Could you check a few things on this model? Use its own coordinates, in mm. A direction names the side the tool comes from. Give positions to 0.01 mm unless a question says otherwise; leave off trailing zeros. Write each loop counter-clockwise with the first axis right and the second up, starting at its lowest first coordinate (ties: lowest second). Pieces come first, ordered by that corner, then holes. Notation, with made-up numbers: (27, 71) -> (82, 71) arc R19 ccw to (82, 90) -> close; hole circle Ø5 at (-35, 45.5). An arc over 180 degrees is marked (long way). One line per question, with ' | ' between items.
from build123d import *

# Parameters (mm, degrees)
ESQUISSE1_W                                  = 4.2
ESQUISSE1_H                                  = 3
ESQUISSE1_W_2                                = 5
ESQUISSE1_H_2                                = 9.7
D_GAGEMENT_M31_D                             = 3.4
ESQUISSE4_W                                  = 1.25
ESQUISSE4_H                                  = 12.7
TROU_POUR_TARAUDAGE_POUR_TROU_TARAUD_2_COUNT = 2
TROU_POUR_TARAUDAGE_POUR_TROU_TARAUD_2_PITCH = 4.6


with BuildPart() as part:
    # Esquisse1 → Révolution1 (revolve)
    with BuildSketch(Plane.XY, mode=Mode.PRIVATE) as r_volution1_sk:
        with Locations((-2.1, 4.5)):
            Rectangle(ESQUISSE1_W, ESQUISSE1_H)
        with Locations((2.5, 7.85)):
            Rectangle(ESQUISSE1_W_2, ESQUISSE1_H_2)
    revolve(r_volution1_sk.sketch.rotate(Axis((0, 0, 0), (1, 0, 0)), 90), axis=Axis((0, 0, 0), (1, 0, 0)))

    # Dégagement M31 (through all)
    with Locations(Plane.ZY):
        with Locations((4.75, 8.227241336), (-4.75, 8.227241336), (-9.5, 0), (-4.75, -8.227241336), (4.75, -8.227241336), (9.5, 0)):
            Hole(D_GAGEMENT_M31_D / 2)

    # Esquisse4 → Trou pour taraudage pour trou taraudé M3x0.51 (revolve, cut)
    with BuildSketch(Plane(origin=(2.5, 0, 0), x_dir=(0, 0, -1), z_dir=(1, 0, 0))):
        with Locations((0.625, 6.35)):
            Rectangle(ESQUISSE4_W, ESQUISSE4_H)
    trou_pour_taraudage_pour_trou_taraud_m3 = revolve(axis=Axis((2.5, -6.35, 0), (0, 1, 0)), mode=Mode.SUBTRACT)

    # Trou pour taraudage pour trou taraud 2: Trou pour taraudage pour trou taraudé M3x0.51 ×2
    with Locations(*[(-i * TROU_POUR_TARAUDAGE_POUR_TROU_TARAUD_2_PITCH, 0, 0) for i in range(1, TROU_POUR_TARAUDAGE_POUR_TROU_TARAUD_2_COUNT)]):
        add(trou_pour_taraudage_pour_trou_taraud_m3, mode=Mode.SUBTRACT)


solid = part.part
Q1. Imagine slicing it at B-B on z = 0. Please give me the cut outline in (x, y), and give its area (4 significant figures).
Answer below:
outline: (-4.2, -6) -> (0, -6) -> (0, -12.7) -> (5, -12.7) -> (5, -3) -> (-4.2, -3) -> close; (-4.2, 3) -> (-3.35, 3) -> (-3.35, 6) -> (-4.2, 6) -> close; (-0.85, 3) -> (1.25, 3) -> (1.25, 12.7) -> (0, 12.7) -> (0, 6) -> (-0.85, 6) -> close; (3.75, 3) -> (5, 3) -> (5, 12.7) -> (3.75, 12.7) -> close | area: 90.45 mm^2
Q2. Will these pins go through, and if not, where does the flat tip stop? pin 1 (1 mm diameter, centred on y = 9.5, z = -2.5, fed in from -X); pin 2 (5 mm diameter, centred on x = 2, y = 7.5, fed in from +Z); pin 3 (2 mm diameter, centred on x = -2.1, z = 0, fed in from +Y); pin 4 (2 mm diameter, centred on y = 8.23, z = 4.75, fed in from -X).
Answer below:
pin 1: stops at x = 0 | pin 2: stops at z = 11.67 | pin 3: stops at y = -2.83 | pin 4: passes through
Q3. Imagine slicing it at C-C on z = -9.5. Please give me the cut outline in (x, y), and give its area (3 significant figures).
Answer below:
outline: (0, -8.43) -> (5, -8.43) -> (5, -1.7) -> (0, -1.7) -> close; (0, 1.7) -> (5, 1.7) -> (5, 8.43) -> (0, 8.43) -> close | area: 67.3 mm^2
Q4. If we mould it in two halves opening along Y, with no side actions, what happens to faces 4 (the cylindrical face through (2.5, 7.7, -10.1)), 5 (the flat face through (-4.2, -3, -1)), 6 (the cylindrical face through (2.5, 6.7, 4))? For each: +Y half, -Y half, draft (parallel to the pull), parting line (faces both ways), or undercut.
Answer below:
face 4: parting line | face 5: draft | face 6: undercut
Q5. If I drill on line 1 along Z through (x, y) = (4, -8); line 2 along Y through (x, z) = (3.4, -4.75); line 3 along Y through (x, z) = (4.25, 6.25), over which ranges is the centre line in solid material (lowest first)?
Answer below:
line 1: z = -9.86 to -6.43, -3.07 to 3.07, 6.43 to 9.86 | line 2: y = -11.78 to -9.93, -6.53 to 6.53, 9.93 to 11.78 | line 3: y = -11.06 to -9.03, -7.43 to 7.43, 9.03 to 11.06
Q6. Imagine slicing it at D-D on x = 2.5. Please give me the cut outline in (y, z), and give its area (3 significant figures).
Answer below:
outline: (2.73, -1.25) arc R3 cw (long way) to (2.73, 1.25) -> (12.64, 1.25) arc R12.7 ccw (long way) to (12.64, -1.25) -> close; hole circle Ø3.4 at (-8.23, -4.75); hole circle Ø3.4 at (-8.23, 4.75); hole circle Ø3.4 at (0, -9.5); hole circle Ø3.4 at (0, 9.5); hole circle Ø3.4 at (8.23, -4.75); hole circle Ø3.4 at (8.23, 4.75) | area: 400 mm^2
Q7. Imagine slicing it at A-A on y = 0. Please give me the cut outline in (x, z), and give its area (3 significant figures).
Answer below:
outline: (-4.2, -6) -> (0, -6) -> (0, -7.8) -> (5, -7.8) -> (5, -3) -> (-4.2, -3) -> close; (-4.2, 3) -> (5, 3) -> (5, 7.8) -> (0, 7.8) -> (0, 6) -> (-4.2, 6) -> close; (0, -12.7) -> (5, -12.7) -> (5, -11.2) -> (0, -11.2) -> close; (0, 11.2) -> (5, 11.2) -> (5, 12.7) -> (0, 12.7) -> close | area: 88.2 mm^2
Q8. On a 3-axis mill with a long thin cutter (end or side, diameter ignored), from which of +Z, -Z, +X, -X, +Y, -Y can I reach the whole of each face in a straight line? I mean faces 1 (the cylindrical face through (2.5, 6.7, -5.5)), 2 (the flat face through (0, 5.5, 3)), 3 (the cylindrical face through (1.26, 7.78, 0.16)). Say none if no direction works.
Answer below:
face 1: +X, -X | face 2: -X | face 3: +Y
